Geometry: final body of the model. Coordinates: model frame, mm. Give positions to 0.01 mm unless a question says otherwise; leave off trailing zeros. Write each loop counter-clockwise with the first axis right and the second up, starting at its lowest first coordinate (ties: lowest second). Pieces come first, ordered by that corner, then holes. Notation, with made-up numbers: (13, 29.25) -> (54, 29.25) arc R9 ccw to (54, 33.25) -> close; hole circle Ø11 at (-39.75, 84.5). An arc over 180 degrees is marked (long way). Answer as a JSON object with one key per item and string values. Group by question number.
(1) Contact query for flat-ended pins moving along their axis: pin 1 Ø2 at (x, z) = (102.5, 4.5) entering from +Y; pin 2 Ø4 at (y, z) = (-71, 1.5) entering from -X; pin 3 Ø5 at (y, z) = (-84, 7.5) entering from +X. Output: stop coordinate, or through.
(2) Section query B-B on x = -83.5. Output: boundary loops of the cut face in (y, z).
(3) Section query A-A on y = -70. Output: boundary loops of the cut face in (x, z).
(4) Material intervals for probe 1 along Z at (x, y) = (30, 13); probe 2 along X at (y, z) = (58.5, 2.5); probe 3 along X at (y, z) = (-30.5, 8.25), sorted ascending.
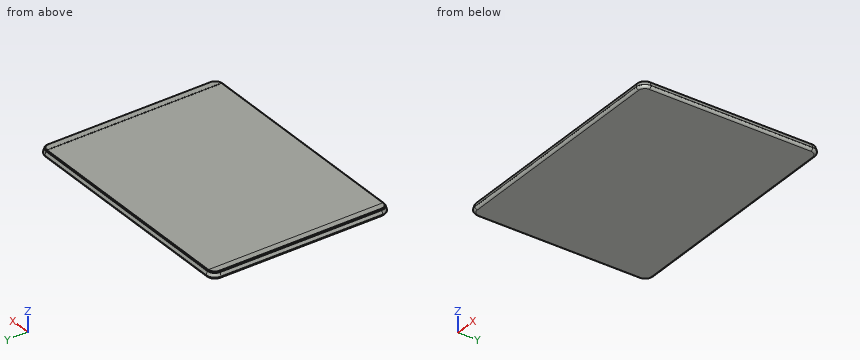
from build123d import *

# Parameters (mm, degrees)
F0_W     = 300
F0_H     = 222
F1_DEPTH = 8.4
F2_R     = 10.6
F3_R     = 3
F4_SIZE2 = 5.3
F4_SIZE  = 1.5
F5_SIZE  = 1
F6_W     = 278.8
F6_H     = 217
F7_DEPTH = 0.1


with BuildPart() as f1:
    # F0 (on Top) → F1 (new body)
    with BuildSketch(Plane.XY):
        Rectangle(F0_W, F0_H)
    extrude(amount=F1_DEPTH)

    # F2
    f2_edges = [f1.edges().sort_by_distance(p)[0] for p in [
        (-150, 111, 4.2),
        (-150, -111, 4.2),
        (150, -111, 4.2),
        (150, 111, 4.2),
    ]]
    fillet(f2_edges, radius=F2_R)

    # F3
    f3_edges = [f1.edges().sort_by_distance(p)[0] for p in [
        (0, 111, 0),
        (146.895332, 107.895332, 0),
        (150, 0, 0),
    ]]
    fillet(f3_edges, radius=F3_R)

    # F4
    f4_edges = [f1.edges().sort_by_distance(p)[0] for p in [
        (-150, 0, 8.4),
        (-146.895332, 107.895332, 8.4),
        (0, 111, 8.4),
    ]]
    f4_side = f1.faces().sort_by_distance((0, 0, 8.4))[0]
    chamfer(f4_edges, length=F4_SIZE, length2=F4_SIZE2, reference=f4_side)

    # F5
    f5_edges = [f1.edges().sort_by_distance(p)[0] for p in [
        (0, 109.5, 8.4),
    ]]
    chamfer(f5_edges, length=F5_SIZE)

    # F6 (on face) → F7 (cut)
    with BuildSketch(Plane.XY.offset(8.4)):
        Rectangle(F6_W, F6_H)
    extrude(amount=-F7_DEPTH, mode=Mode.SUBTRACT)


solid = f1.part
Answer list:
{
 "1": {"pin 1": "y = 110.89", "pin 2": "x = -150", "pin 3": "x = 149.46"},
 "2": {"outline": "(-111, 3) arc R3 ccw to (-108, 0) -> (108, 0) arc R3 ccw to (111, 3) -> (111, 3.1) -> (109.77, 7.44) -> (108.5, 8.4) -> (108.5, 8.3) -> (-108.5, 8.3) -> (-108.5, 8.4) -> (-109.77, 7.44) -> (-111, 3.1) -> close"},
 "3": {"outline": "(-150, 3) arc R3 ccw to (-147, 0) -> (147, 0) arc R3 ccw to (150, 3) -> (150, 3.1) -> (148.77, 7.44) -> (147.5, 8.4) -> (139.4, 8.4) -> (139.4, 8.3) -> (-139.4, 8.3) -> (-139.4, 8.4) -> (-147.5, 8.4) -> (-148.77, 7.44) -> (-150, 3.1) -> close"},
 "4": {"probe 1": "0 to 8.3", "probe 2": "-149.96 to 149.96", "probe 3": "-147.7 to 147.7"}
}
